CAD build for the part. Positions are in the model's coordinates, mm. A direction names the side the tool comes from. Give positions to 0.01 mm unless a question says otherwise; leave off trailing zeros. Order: outer loops, then holes, each group sorted by start corner. A loop starts at its lowest first (then second) coordinate and runs counter-clockwise, first axis right, second up.
Item 1: Two-plate mould, pull along Y, no slides. Class faces 1 (the cylindrical face through (-1.734, 2.594, 2.262)), 2 (the cylindrical face through (-2.44, -14.51, 0.54)), 3 (the flat face through (0, 40, 0)): released by +Y, released by -Y, zero draft, split by the parting line, or undercut.
Item 2: Wall check: L1, parallel to Z at x = -0.1, y = 15; L2, parallel to Z at x = 1.35, y = 30. Give the ranges that are in metal, low to high.
Item 3: Which spindle directions (+Z, -Z, +X, -X, +Y, -Y) get a long thin tool onto all of the face, cutting with end or side? Do faces 4 (the flat face through (2, -14, 2)), 5 (the cylindrical face through (-1.734, 37.194, 2.262)), 6 (the cylindrical face through (0.9, 19.66, 2.86)). Say none if no direction does.
Item 4: Flat gauge pin, fed straight in: P1, Ø2, axis at x = 1.5, y = 12.5, coming from the +Z side. Where does the tip first touch, or does it go through?
Item 5: Band-saw the part on A-A on y = -9. Give the cut face in (x, z), plus the area to 3 significant figures.
```python
from build123d import *

# Parameters (mm, degrees)
SKETCH1_R           = 3
BOSS_EXTRUDE1_DEPTH = 40
CUT_EXTRUDE1_START  = 3.2
SKETCH2_R           = 3
SKETCH2_R_2         = 2.85
CUT_EXTRUDE1_DEPTH  = 0.8
CUT_EXTRUDE2_START  = -2.2
SKETCH3_R           = 3
SKETCH3_R_2         = 2.85
CUT_EXTRUDE2_DEPTH  = 0.8
CHAMFER1_SIZE       = 0.5
BOSS_EXTRUDE2_START = 15
SKETCH4_R           = 3
BOSS_EXTRUDE2_DEPTH = 15
SKETCH5_R           = 3
SKETCH5_R_2         = 2.5
CUT_EXTRUDE3_DEPTH  = 1


with BuildPart() as part:
    # Sketch1 → Boss-Extrude1 (new body)
    with BuildSketch(Plane(origin=(0, 0, 0), x_dir=(1, 0, 0), z_dir=(0, 1, 0))):
        with Locations(Location((0, 0, 0), (0, 0, 270))):
            Circle(SKETCH1_R)
    extrude(amount=BOSS_EXTRUDE1_DEPTH)

    # Sketch2 → Cut-Extrude1 (cut)
    with BuildSketch(Plane.XZ.offset(-40).offset(CUT_EXTRUDE1_START)):
        with Locations(Location((0, 0, 0), (0, 0, 270))):
            Circle(SKETCH2_R)
        with Locations(Location((0, 0, 0), (0, 0, 270))):
            Circle(SKETCH2_R_2, mode=Mode.SUBTRACT)
    extrude(amount=-CUT_EXTRUDE1_DEPTH, mode=Mode.SUBTRACT)

    # Sketch3 → Cut-Extrude2 (cut)
    with BuildSketch(Plane.XZ.offset(CUT_EXTRUDE2_START)):
        with Locations(Location((0, 0, 0), (0, 0, 270))):
            Circle(SKETCH3_R)
        with Locations(Location((0, 0, 0), (0, 0, 270))):
            Circle(SKETCH3_R_2, mode=Mode.SUBTRACT)
    extrude(amount=-CUT_EXTRUDE2_DEPTH, mode=Mode.SUBTRACT)

    # Chamfer1
    chamfer1_edges = [part.edges().sort_by_distance(p)[0] for p in [
        (0, 40, -3),
    ]]
    chamfer(chamfer1_edges, length=CHAMFER1_SIZE)

    # Sketch4 → Boss-Extrude2 (add)
    with BuildSketch(Plane.XZ.offset(BOSS_EXTRUDE2_START)):
        with Locations(Location((0, 0, 0), (0, 0, 270))):
            Circle(SKETCH4_R)
    extrude(amount=-BOSS_EXTRUDE2_DEPTH)

    # Sketch5 → Cut-Extrude3 (cut)
    with BuildSketch(Plane.XZ.offset(15)):
        with Locations(Location((0, 0, 0), (0, 0, 270))):
            Circle(SKETCH5_R)
        with Locations(Location((0, 0, 0), (0, 0, 270))):
            Circle(SKETCH5_R_2, mode=Mode.SUBTRACT)
    extrude(amount=-CUT_EXTRUDE3_DEPTH, mode=Mode.SUBTRACT)


solid = part.part
```
The answers:
1. face 1: undercut
1. face 2: zero draft
1. face 3: released by +Y
2. L1: z = -3 to 3
2. L2: z = -2.68 to 2.68
3. face 4: -Y
3. face 5: none
3. face 6: +Y, -Y
4. P1: stops at z = 2.96
5. outline: circle Ø6 at (0, 0)
5. area: 28.3 mm2
